from build123d import *

# Parameters (mm, degrees)
F1_DEPTH = 5.08
F2_R     = 4


# Not quite as in the source:
# - a feature names something its author has since deleted; it is built from what else it names


with BuildPart() as f1:
    # F0 (on Top) → F1 (new body)
    with BuildSketch(Plane.XY):
        with BuildLine():
            Line((10.9156670719, 55.8519247654), (-50.5843329281, 55.8519247654))
            ThreePointArc((-50.5843329281, 55.8519247654), (-50.7903791398, 55.0931866065), (-51.3519110531, 54.5428952787))
            Line((-51.3519110531, 54.5428952787), (-49.566514597, 51.3519247654))
            Line((-49.566514597, 51.3519247654), (-11.1088099211, 51.3519247654))
            Line((-11.1088099211, 51.3519247654), (-3.1543997556, 51.3519247654))
            Line((-3.1543997556, 51.3519247654), (5.4156670719, 51.3519247654))
            Line((5.4156670719, 51.3519247654), (10.9156670719, 51.3519247654))
            Line((10.9156670719, 51.3519247654), (10.9156670719, 55.8519247654))
        make_face()
        with BuildLine():
            Line((-11.1088099211, 4.5), (-23.3521512592, 4.5))
            Line((-23.3521512592, 4.5), (-21.5667548031, 1.3090294867))
            ThreePointArc((-21.5667548031, 1.3090294867), (-20.0755947692, 1.2939537883), (-19.3343329281, 0))
            Line((-19.3343329281, 0), (10.9156670719, 0))
            Line((10.9156670719, 0), (10.9156670719, 4.5))
            Line((10.9156670719, 4.5), (5.4156670719, 4.5))
            Line((5.4156670719, 4.5), (-3.1543997556, 4.5))
            Line((-3.1543997556, 4.5), (-11.1088099211, 4.5))
        make_face()
        with BuildLine():
            ThreePointArc((-51.3519110531, 54.5428952787), (-53.3782867164, 56.6106629243), (-50.5843329281, 55.8519247654))
            Line((-50.5843329281, 55.8519247654), (10.9156670719, 55.8519247654))
            Line((10.9156670719, 55.8519247654), (71.6656670719, 55.8519247654))
            ThreePointArc((71.6656670719, 55.8519247654), (73.9156670719, 58.1019247654), (76.1656670719, 55.8519247654))
            ThreePointArc((76.1656670719, 55.8519247654), (75.0537743102, 53.910994083), (72.8170342594, 53.8883805354))
            Line((72.8170342594, 53.8883805354), (71.3978487408, 51.3519247654))
            Line((71.3978487408, 51.3519247654), (81.8841302488, 51.3519247654))
            Line((81.8841302488, 51.3519247654), (81.8841302488, 60.3519247654))
            Line((81.8841302488, 60.3519247654), (-60.052796105, 60.3519247654))
            Line((-60.052796105, 60.3519247654), (-60.052796105, 51.3519247654))
            Line((-60.052796105, 51.3519247654), (-49.566514597, 51.3519247654))
            Line((-49.566514597, 51.3519247654), (-51.3519110531, 54.5428952787))
        make_face()
        with BuildLine():
            Line((-21.5667548031, 1.3090294867), (-23.3521512592, 4.5))
            Line((-23.3521512592, 4.5), (-27.3365851734, 4.5))
            Line((-27.3365851734, 4.5), (-27.3365851734, -4.5))
            Line((-27.3365851734, -4.5), (49.1679193172, -4.5))
            Line((49.1679193172, -4.5), (49.1679193172, 4.5))
            Line((49.1679193172, 4.5), (45.183485403, 4.5))
            Line((45.183485403, 4.5), (43.3980889469, 1.3090294867))
            ThreePointArc((43.3980889469, 1.3090294867), (43.9596208602, 0.7587381589), (44.1656670719, 0))
            ThreePointArc((44.1656670719, 0), (42.6656670719, -1.5), (41.1656670719, 0))
            Line((41.1656670719, 0), (10.9156670719, 0))
            Line((10.9156670719, 0), (-19.3343329281, 0))
            ThreePointArc((-19.3343329281, 0), (-21.593071087, -1.2939537883), (-21.5667548031, 1.3090294867))
        make_face()
        with BuildLine():
            Line((16.4156670719, 4.5), (10.9156670719, 4.5))
            Line((10.9156670719, 4.5), (10.9156670719, 0))
            Line((10.9156670719, 0), (41.1656670719, 0))
            ThreePointArc((41.1656670719, 0), (41.906928913, 1.2939537883), (43.3980889469, 1.3090294867))
            Line((43.3980889469, 1.3090294867), (45.183485403, 4.5))
            Line((45.183485403, 4.5), (32.9401440649, 4.5))
            Line((32.9401440649, 4.5), (24.9857338994, 4.5))
            Line((24.9857338994, 4.5), (16.4156670719, 4.5))
        make_face()
        with BuildLine():
            Line((71.6656670719, 55.8519247654), (10.9156670719, 55.8519247654))
            Line((10.9156670719, 55.8519247654), (10.9156670719, 51.3519247654))
            Line((10.9156670719, 51.3519247654), (16.4156670719, 51.3519247654))
            Line((16.4156670719, 51.3519247654), (24.9857338994, 51.3519247654))
            Line((24.9857338994, 51.3519247654), (32.9401440649, 51.3519247654))
            Line((32.9401440649, 51.3519247654), (71.3978487408, 51.3519247654))
            Line((71.3978487408, 51.3519247654), (72.8170342594, 53.8883805354))
            ThreePointArc((72.8170342594, 53.8883805354), (71.9747363894, 54.7138175271), (71.6656670719, 55.8519247654))
        make_face()
        Polygon((10.9156670719, 27.9259623827), (10.9156670719, 51.3519247654), (5.4156670719, 51.3519247654), (5.4156670719, 39.2025500407), (5.4156670719, 27.9259623827), align=None)
        Polygon((10.9156670719, 4.5), (10.9156670719, 27.9259623827), (5.4156670719, 27.9259623827), (5.4156670719, 16.6493747247), (5.4156670719, 4.5), align=None)
        Polygon((16.4156670719, 51.3519247654), (10.9156670719, 51.3519247654), (10.9156670719, 27.9259623827), (16.4156670719, 27.9259623827), (16.4156670719, 39.2025500407), align=None)
        Polygon((16.4156670719, 27.9259623827), (10.9156670719, 27.9259623827), (10.9156670719, 4.5), (16.4156670719, 4.5), (16.4156670719, 16.6493747247), align=None)
        Polygon((-3.1543997556, 51.3519247654), (-11.1088099211, 51.3519247654), (5.4156670719, 27.9259623827), (5.4156670719, 39.2025500407), align=None)
        Polygon((5.4156670719, 27.9259623827), (-11.1088099211, 4.5), (-3.1543997556, 4.5), (5.4156670719, 16.6493747247), align=None)
        Polygon((32.9401440649, 4.5), (16.4156670719, 27.9259623827), (16.4156670719, 16.6493747247), (24.9857338994, 4.5), align=None)
        Polygon((16.4156670719, 39.2025500407), (16.4156670719, 27.9259623827), (32.9401440649, 51.3519247654), (24.9857338994, 51.3519247654), align=None)
    extrude(amount=F1_DEPTH)

    # F2
    f2_edges = [f1.edges().sort_by_distance(p)[0] for p in [
        (-60.052796, 60.351925, 2.54),
        (-60.052796, 51.351925, 2.54),
        (81.88413, 60.351925, 2.54),
        (81.88413, 51.351925, 2.54),
        (49.167919, 4.5, 2.54),
        (49.167919, -4.5, 2.54),
        (-27.336585, 4.5, 2.54),
        (-27.336585, -4.5, 2.54),
    ]]
    fillet(f2_edges, radius=F2_R)


solid = f1.part
Input: part model. Units: mm. Frame: model coordinates. A direction names the side the tool comes from. Give positions to 0.01 mm unless a question says otherwise; leave off trailing zeros. Loops run counter-clockwise (first coordinate to the right, second up) from the corner with the lowest first, then second, coordinate; pieces in that order, holes last. Notation, with made-up numbers: M 18,38.5 L 67,38.5 A24 ccw 67,51.5 Z; hole C 86,-11 d4. An arc over 180 degrees is marked long. Use one line per item in the form item = value.
1. Section query C-C, the plane z = 0.8. Count the separate pieces of the cut face and the enclosed holes in it, and give its area (3 significant figures).
Numbers:
separate_pieces = 1
enclosed_holes = 8
area = 2,980 mm²
2. Section query A-A, the plane y = 46. Return the cut outline in (x, z).
Numbers:
outline = M -7.33,0 L 0.62,0 L 0.62,5.08 L -7.33,5.08 Z; M 5.42,0 L 16.42,0 L 16.42,5.08 L 5.42,5.08 Z; M 21.21,0 L 29.16,0 L 29.16,5.08 L 21.21,5.08 Z
3. Reachability of faces 4 (the face through (20.64, 10.66, 2.5)), 5 (the face through (-17, 4.5, 3)), 6 (the face through (24.794, 16.049, 2.504)) from +Z, -Z, +X, -X, +Y, -Y: full face, straight path, thin tool, end or side. Return the list, or none.
Numbers:
face_4 = +Z, -Z
face_5 = +Z, -Z, -X
face_6 = +Z, -Z, +X
4. Line query: L1, parallel to Y at x = -17.5, z = 3.75; L2, parallel to X at y = 16, z = 1.45; L3, parallel to Y at x = 43, z = 2.7. Output: solid intervals per line, ascending.
Numbers:
L1 = -4.5 to 4.5, 51.35 to 60.35
L2 = -3 to 4.96, 5.42 to 16.42, 16.87 to 24.83
L3 = -4.5 to -1.46, 1.46 to 4.5, 51.35 to 60.35
5. Section query B-B, the plane x = 20. Return the cut outline in (y, z).
Numbers:
outline = M -4.5,0 L 4.5,0 L 4.5,5.08 L -4.5,5.08 Z; M 11.57,0 L 22.84,0 L 22.84,5.08 L 11.57,5.08 Z; M 33.01,0 L 44.28,0 L 44.28,5.08 L 33.01,5.08 Z; M 51.35,0 L 60.35,0 L 60.35,5.08 L 51.35,5.08 Z
6. First-contact query: pin 1 (0.5 mm diameter, centred on y = 0, z = 1.5, fed in from -X); pin 2 (6 mm diameter, centred on x = 4, y = 53.5, fed in from -Z); pin 3 (1.5 mm diameter, centred on x = -30.5, z = 2.5, fed in from -Y); pin 4 (1.5 mm diameter, centred on y = 11, z = 3.5, fed in from -X). Flat tips, straight axial feed; report the tip coordinate or a pass-through.
Numbers:
pin_1 = -27.34
pin_2 = 0
pin_3 = 51.35
pin_4 = -7.05
7. Pull-direction query (X, two-part tool) for faces 1 (the face through (39, 4.5, 3)), 2 (the face through (21, 4.5, 3)), 3 (the face through (48.027, 3.297, 2.576)); classes: released by +X, released by -X, zero draft, split by the parting line, or undercut.
Numbers:
face_1 = zero draft
face_2 = undercut
face_3 = released by +X
8. Section query D-D, the plane x = 58.5. Return the cut outline in (y, z), and give its area (3 significant figures).
Numbers:
outline = M 51.35,0 L 60.35,0 L 60.35,5.08 L 51.35,5.08 Z
area = 45.7 mm²
